Print and shaded views of the part. All mm, measured from the part's lowest x, y and z. Round coordinates to 2 decimals unless told otherwise and drop trailing zeros. Order: outer loops, then holes, each group sorted by start corner. A loop starts at its lowest first (then second) coordinate and runs counter-clockwise, first axis right, second up.
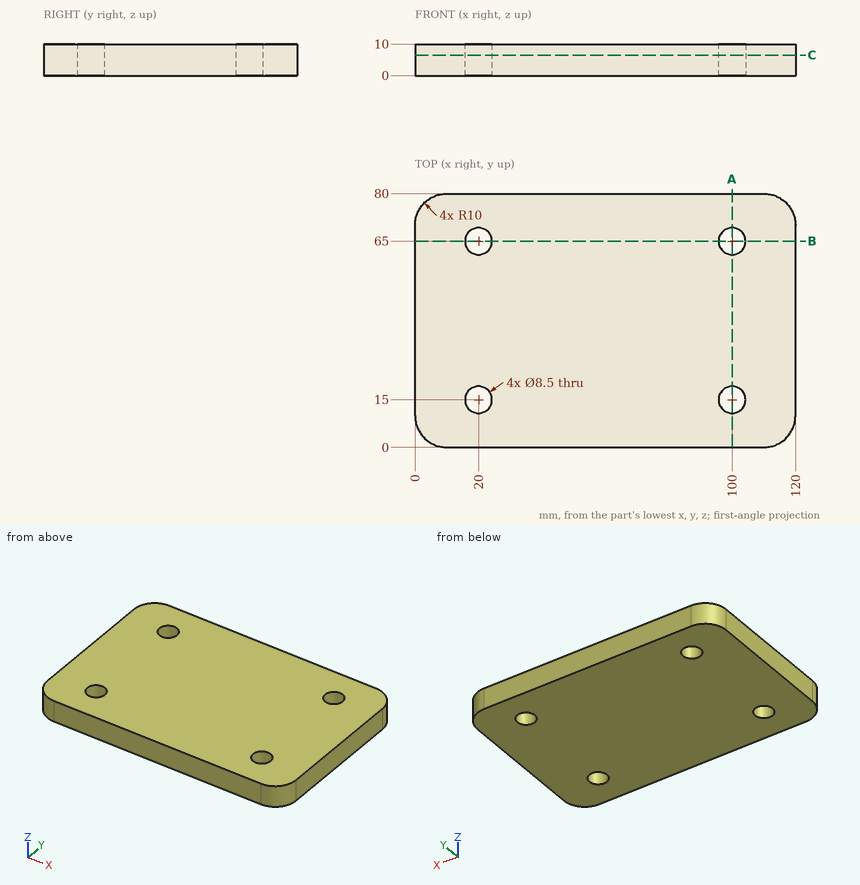
1. Drill centre lines: line 1 (Y direction, x = 20, z = 4.5); line 2 (X direction, y = 66.5, z = 5.75); line 3 (X direction, y = 17.5, z = 0.75). Where is each one in solid material? Low to high.
2. Cut at B-B, the plane y = 65. Write the cut outline in (x, z), and give its area (3 significant figures).
3. Cut at C-C, the plane z = 6.5. Write the cut outline in (x, y), and give its area (3 significant figures).
4. Cut at A-A, the plane x = 100. Write the cut outline in (y, z), and give its area (3 significant figures).
Outcome:
1. line 1: y = 0 to 10.75, 19.25 to 60.75, 69.25 to 80
1. line 2: x = 0 to 16.02, 23.98 to 96.02, 103.98 to 120
1. line 3: x = 0 to 16.56, 23.44 to 96.56, 103.44 to 120
2. outline: (0, 0) - (15.75, 0) - (15.75, 10) - (0, 10) - close; (24.25, 0) - (95.75, 0) - (95.75, 10) - (24.25, 10) - close; (104.25, 0) - (120, 0) - (120, 10) - (104.25, 10) - close
2. area: 1,030 mm2
3. outline: (0, 10) arc R10 ccw to (10, 0) - (110, 0) arc R10 ccw to (120, 10) - (120, 70) arc R10 ccw to (110, 80) - (10, 80) arc R10 ccw to (0, 70) - close; hole circle Ø8.5 at (20, 15); hole circle Ø8.5 at (20, 65); hole circle Ø8.5 at (100, 15); hole circle Ø8.5 at (100, 65)
3. area: 9,290 mm2
4. outline: (0, 0) - (10.75, 0) - (10.75, 10) - (0, 10) - close; (19.25, 0) - (60.75, 0) - (60.75, 10) - (19.25, 10) - close; (69.25, 0) - (80, 0) - (80, 10) - (69.25, 10) - close
4. area: 630 mm2
